from build123d import *

# Parameters (mm, degrees)
SKETCH1_R          = 62.5
SKETCH1_R_2        = 42.5
BODY_DEPTH         = 5
SKETCH2_R          = 4
CUT_EXTRUDE1_DEPTH = 11
HOLES_COUNT        = 6


with BuildPart() as part:
    # Sketch1 → Body (new body, symmetric)
    with BuildSketch(Plane.XY):
        Circle(SKETCH1_R)
        Circle(SKETCH1_R_2, mode=Mode.SUBTRACT)
    extrude(amount=BODY_DEPTH, both=True)

    # Sketch2 → Cut-Extrude1 (cut, through all)
    with BuildSketch(Plane.XY.offset(5)):
        with Locations((0, 52.5)):
            Circle(SKETCH2_R)
    cut_extrude1 = extrude(amount=-CUT_EXTRUDE1_DEPTH, mode=Mode.SUBTRACT)

    # Holes: Cut-Extrude1 ×6 about axis
    holes_axis = Axis((0, 0, 0), (0, 0, 1))
    for i in range(1, HOLES_COUNT):
        add(cut_extrude1.rotate(holes_axis, i * 360 / HOLES_COUNT), mode=Mode.SUBTRACT)


solid = part.part
Could you check a few things on this model? Use its own coordinates, in mm. Give positions to 0.01 mm unless a question says otherwise; leave off trailing zeros. Loops run counter-clockwise (first coordinate to the right, second up) from the corner with the lowest first, then second, coordinate; pieces in that order, holes last. Notation, with made-up numbers: (-33, 0.5) -> (4, 0.5) arc R37 ccw to (4, 39.5) -> close; hole circle Ø6 at (45, 68). An arc over 180 degrees is marked (long way). Return JSON: item names as keys, results as strings.
Item 1: I need wall thicknesses on L1, parallel to Y at x = 0, z = 2.75; L2, parallel to X at y = -26.5, z = 2.5; L3, parallel to Y at x = 46, z = 3.5. Which ranges of each line are inside material? Lowest first, please. Write a range as from..to.
Geometry results:
{"L1": "y = -62.5..-56.5, -48.5..-42.5, 42.5..48.5, 56.5..62.5", "L2": "x = -56.6..-49.46, -41.47..-33.23, 33.23..41.47, 49.46..56.6", "L3": "y = -42.31..-30.21, -22.29..22.29, 30.21..42.31"}
Item 2: I'm going to push flat-ended pins straight in: pin 1 (5 mm diameter, centred on y = -13.5, z = -1, fed in from -X); pin 2 (6 mm diameter, centred on x = -40.5, z = -0.5, fed in from +Y); pin 3 (3 mm diameter, centred on x = 27, z = 0.5, fed in from -Y). Where does each tip first touch, or does it pass through?
Geometry results:
{"pin 1": "stops at x = -61.52", "pin 2": "stops at y = 50", "pin 3": "stops at y = -57.06"}
Item 3: If we section it at B-B on y = 0: List the corners of the cut face in (x, z) for me, plus the area to 3 significant figures.
Geometry results:
{"outline": "(-62.5, -5) -> (-42.5, -5) -> (-42.5, 5) -> (-62.5, 5) -> close; (42.5, -5) -> (62.5, -5) -> (62.5, 5) -> (42.5, 5) -> close", "area": "400 mm²"}
Item 4: If we section it at D-D on x = -21.5: List the corners of the cut face in (y, z) for me.
Geometry results:
{"outline": "(-58.69, -5) -> (-36.66, -5) -> (-36.66, 5) -> (-58.69, 5) -> close; (36.66, -5) -> (58.69, -5) -> (58.69, 5) -> (36.66, 5) -> close"}
Item 5: If we section it at C-C on y = -28: List the corners of the cut face in (x, z) for me.
Geometry results:
{"outline": "(-55.88, -5) -> (-49.06, -5) -> (-49.06, 5) -> (-55.88, 5) -> close; (-41.87, -5) -> (-31.97, -5) -> (-31.97, 5) -> (-41.87, 5) -> close; (31.97, -5) -> (41.87, -5) -> (41.87, 5) -> (31.97, 5) -> close; (49.06, -5) -> (55.88, -5) -> (55.88, 5) -> (49.06, 5) -> close"}
Item 6: If we section it at A-A on x = 0: List the corners of the cut face in (y, z) for me, plus the area to 3 significant figures.
Geometry results:
{"outline": "(-62.5, -5) -> (-56.5, -5) -> (-56.5, 5) -> (-62.5, 5) -> close; (-48.5, -5) -> (-42.5, -5) -> (-42.5, 5) -> (-48.5, 5) -> close; (42.5, -5) -> (48.5, -5) -> (48.5, 5) -> (42.5, 5) -> close; (56.5, -5) -> (62.5, -5) -> (62.5, 5) -> (56.5, 5) -> close", "area": "240 mm²"}
Item 7: We'd pull the mould along Y, two halves only. Please class faces 1 (the cylindrical face through (-62.44, 2.75, 0.07)), 2 (the cylindrical face through (0.867, -48.595, 0.07)), 3 (the flat face through (41, -13, 5)): +Y half, -Y half, draft (parallel to the pull), parting line (faces both ways), or undercut.
Geometry results:
{"face 1": "parting line", "face 2": "undercut", "face 3": "draft"}
